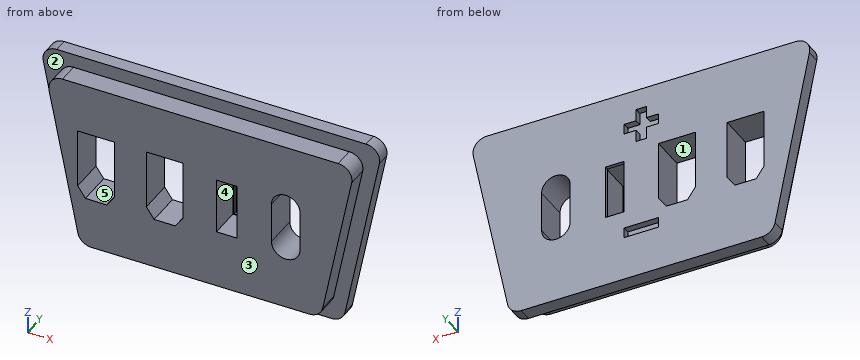
from build123d import *

# Parameters (mm, degrees)
BOSS_EXTRUDE1_DEPTH = 3
BOSS_EXTRUDE2_DEPTH = 2
FILLET1_R           = 2
CUT_EXTRUDE1_DEPTH  = 5
LPATTERN1_COUNT     = 2
LPATTERN1_PITCH     = 10
SKETCH5_W           = 2.7
SKETCH5_H           = 7.9
CUT_EXTRUDE2_DEPTH  = 5
SKETCH6_W           = 3
SKETCH6_H           = 8.1
CUT_EXTRUDE3_DEPTH  = 4.5
USB_C_HOLE_DEPTH    = 5
SKETCH8_W           = 1.75
SKETCH8_H           = 1.5
SKETCH8_W_2         = 1.5
SKETCH8_H_2         = 1.75
SKETCH8_W_3         = 5
POSNEGSIGNS_DEPTH   = 1


with BuildPart() as part:
    # Sketch1 → Boss-Extrude1 (new body)
    with BuildSketch(Plane(origin=(0, 0, 0), x_dir=(1, 0, 0), z_dir=(0, 1, 0))):
        Polygon((-17.5, 12.5), (17.5, 12.5), (22.5, -12.5), (-22.5, -12.5), align=None)
    extrude(amount=BOSS_EXTRUDE1_DEPTH)

    # Sketch2 → Boss-Extrude2 (add)
    with BuildSketch(Plane(origin=(0, 3, 0), x_dir=(1, 0, 0), z_dir=(0, 1, 0))):
        Polygon((-19.139607805, 14.5), (19.139607805, 14.5), (24.939607805, -14.5), (-24.939607805, -14.5), align=None)
    extrude(amount=BOSS_EXTRUDE2_DEPTH)

    # Fillet1
    fillet1_edges = [part.edges().sort_by_distance(p)[0] for p in [
        (-19.139607805, 4, -14.5),
        (-24.939607805, 4, 14.5),
        (24.939607805, 4, 14.5),
        (19.139607805, 4, -14.5),
        (-17.5, 1.5, -12.5),
        (17.5, 1.5, -12.5),
        (22.5, 1.5, 12.5),
        (-22.5, 1.5, 12.5),
    ]]
    fillet(fillet1_edges, radius=FILLET1_R)

    # Sketch3 → Cut-Extrude1 (cut)
    with BuildSketch(Plane(origin=(0, 5, 0), x_dir=(1, 0, 0), z_dir=(0, 1, 0))):
        Polygon((-7.85, -5.1), (-2.5, -5.1), (-2.5, 3.5), (-3.625, 5.1), (-6.725, 5.1), (-7.85, 3.5), align=None)
    cut_extrude1 = extrude(amount=-CUT_EXTRUDE1_DEPTH, mode=Mode.SUBTRACT)

    # LPattern1: Cut-Extrude1 ×2
    with Locations(*[(-i * LPATTERN1_PITCH, 0, 0) for i in range(1, LPATTERN1_COUNT)]):
        add(cut_extrude1, mode=Mode.SUBTRACT)

    # Sketch5 → Cut-Extrude2 (cut)
    with BuildSketch(Plane.XZ):
        with Locations((3.85, 0)):
            Rectangle(SKETCH5_W, SKETCH5_H)
    extrude(amount=-CUT_EXTRUDE2_DEPTH, mode=Mode.SUBTRACT)

    # Sketch6 → Cut-Extrude3 (cut)
    with BuildSketch(Plane.XZ):
        with Locations((3.85, 0)):
            Rectangle(SKETCH6_W, SKETCH6_H)
    extrude(amount=-CUT_EXTRUDE3_DEPTH, mode=Mode.SUBTRACT)

    # Sketch7 → USB-C Hole (cut)
    with BuildSketch(Plane.XZ):
        with BuildLine():
            Line((14.51, 2.92), (14.51, -2.92))
            ThreePointArc((14.51, -2.92), (12.43, -5), (10.35, -2.92))
            Line((10.35, -2.92), (10.35, 2.92))
            ThreePointArc((10.35, 2.92), (12.43, 5), (14.51, 2.92))
        make_face()
    extrude(amount=-USB_C_HOLE_DEPTH, mode=Mode.SUBTRACT)

    # Sketch8 → PosNegSigns (cut)
    with BuildSketch(Plane(origin=(0, 5, 0), x_dir=(1, 0, 0), z_dir=(0, 1, 0))):
        with Locations((-1.625, -9)):
            Rectangle(SKETCH8_W, SKETCH8_H)
        with Locations((0, -10.625)):
            Rectangle(SKETCH8_W_2, SKETCH8_H_2)
        with Locations((0, -9)):
            Rectangle(SKETCH8_W_2, SKETCH8_H)
        with Locations((1.625, -9)):
            Rectangle(SKETCH8_W, SKETCH8_H)
        with Locations((0, -7.375)):
            Rectangle(SKETCH8_W_2, SKETCH8_H_2)
        with Locations((0, 7.25)):
            Rectangle(SKETCH8_W_3, SKETCH8_H)
    extrude(amount=-POSNEGSIGNS_DEPTH, mode=Mode.SUBTRACT)


solid = part.part
Model file for the job. Use its own axes, mm. Face numbers are marked on the shaded views. A direction names the side the tool comes from. Round coordinates to 2 decimals unless told otherwise and drop trailing zeros. Loops run counter-clockwise (first coordinate to the right, second up) from the corner with the lowest first, then second, coordinate; pieces in that order, holes last.
1. Wall check: probe 1 along X at (y, z) = (1.45, -3); probe 2 along Z at (x, y) = (-16, 0.95); probe 3 along X at (y, z) = (0.55, -3.75). Give the ranges that are in metal, low to high.
Check values:
probe 1: x = -19.4 to -17.85, -12.5 to -7.85, -2.5 to 2.35, 5.35 to 10.35, 14.51 to 19.4
probe 2: z = -12.5 to -5.1, 5.1 to 12.5
probe 3: x = -19.25 to -17.67, -12.68 to -7.67, -2.68 to 2.35, 5.35 to 10.52, 14.34 to 19.25
2. Tool access for the marked faces 3, 4 and 5: list every direction of +Z, -Z, +X, -X, +Y, -Y with a clear straight run to the whole face (end or side of a thin tool).
Check values:
face 3: +Z, -Z, +X, -X, -Y
face 4: -Y
face 5: +Y, -Y
3. Mould opens along X. For the marked faces 1 and 2 say: +X half, -X half, draft (parallel to the pull), parting line (faces both ways), or undercut.
Check values:
face 1: undercut
face 2: draft
4. Band-saw the part on B-B, the plane x = -5.5. List the corners of the cut face in (y, z).
Check values:
outline: (0, -12.5) - (3, -12.5) - (3, -14.5) - (5, -14.5) - (5, -5.1) - (0, -5.1) - close; (0, 5.1) - (5, 5.1) - (5, 14.5) - (3, 14.5) - (3, 12.5) - (0, 12.5) - close
5. Drop flat-ended pins along their axis: P1, Ø1.5, axis at x = -5, y = 2, coming from the +Z side; P2, Ø0.8, axis at y = 4.5, z = -7, coming from the -X side; P3, Ø1.3, axis at y = 3, z = -1, coming from the +X side. Give the stop position or say it passes through.
Check values:
P1: stops at z = 12.5
P2: stops at x = -20.72
P3: stops at x = 21.97
6. Band-saw the part on D-D, the plane x = -12. List the corners of the cut face in (y, z), and give its area (3 significant figures).
Check values:
outline: (0, -12.5) - (3, -12.5) - (3, -14.5) - (5, -14.5) - (5, 14.5) - (3, 14.5) - (3, 12.5) - (0, 12.5) - close
area: 133 mm2
7. Band-saw the part on C-C, the plane z = 0.75. List the corners of the cut face in (x, y).
Check values:
outline: (-22.19, 3) - (-20.15, 3) - (-20.15, 0) - (-17.85, 0) - (-17.85, 5) - (-22.19, 5) - close; (-12.5, 0) - (-7.85, 0) - (-7.85, 5) - (-12.5, 5) - close; (-2.5, 0) - (2.35, 0) - (2.35, 4.5) - (2.5, 4.5) - (2.5, 5) - (-2.5, 5) - close; (5.2, 4.5) - (5.35, 4.5) - (5.35, 0) - (10.35, 0) - (10.35, 5) - (5.2, 5) - close; (14.51, 0) - (20.15, 0) - (20.15, 3) - (22.19, 3) - (22.19, 5) - (14.51, 5) - close
8. Band-saw the part on A-A, the plane y = 3.5. List the corners of the cut face in (x, z) (3 decimals), and give its area (3 significant figures).
Check values:
outline: (-24.461, 12.108) - (-19.461, -12.892) arc R2 ccw to (-17.5, -14.5) - (17.5, -14.5) arc R2 ccw to (19.461, -12.892) - (24.461, 12.108) arc R2 ccw to (22.5, 14.5) - (-22.5, 14.5) arc R2 ccw to start; hole (-17.85, -3.5) - (-16.725, -5.1) - (-13.625, -5.1) - (-12.5, -3.5) - (-12.5, 5.1) - (-17.85, 5.1) - close; hole (-7.85, -3.5) - (-6.725, -5.1) - (-3.625, -5.1) - (-2.5, -3.5) - (-2.5, 5.1) - (-7.85, 5.1) - close; hole (2.35, -4.05) - (5.35, -4.05) - (5.35, 4.05) - (2.35, 4.05) - close; hole (10.35, -2.92) arc R2.08 ccw to (14.51, -2.92) - (14.51, 2.92) arc R2.08 ccw to (10.35, 2.92) - close
area: 1,110 mm2
